Here's how the part is built. I have some questions about the finished solid (model axes, mm). A direction names the side the tool comes from. Round coordinates to 2 decimals unless told otherwise and drop trailing zeros. Write each loop counter-clockwise with the first axis right and the second up, starting at its lowest first coordinate (ties: lowest second). Pieces come first, ordered by that corner, then holes. Notation, with made-up numbers: M 31.25,28.5 L 89.25,28.5 A30 ccw 89.25,53.5 Z; hole C 3,26 d9. An arc over 180 degrees is marked long. Use a Markdown table: item, result. Add a question column.
Autodesk Inventor part; units mm, degrees
ref_plane "YZ Plane" through (0, 0, 0) normal (1, 0, 0) x (0, 1, 0)
ref_plane "XZ Plane" through (0, 0, 0) normal (0, 1, 0) x (-1, 0, 0)
ref_plane "XY Plane" through (0, 0, 0) normal (0, 0, 1) x (1, 0, 0)
sketch "main" plane through (0, 0, 0) normal (0, 0, 1) x (1, 0, 0)
  circle A0 centre (-11.2144, -104.2473) radius 2.1844
  circle A1 centre (1.4856, -104.2473) radius 2.1844
  circle A2 centre (48.9096, 6.9894) radius 2.1844
  circle A3 centre (-26.5889, 92.8058) radius 2.1844
  arc A4 (1.4856, -110.5973) -> (7.2979, -106.8047) centre (1.4856, -104.2473) ccw
  arc A5 (-17.0266, -101.6899) -> (-11.2144, -110.5973) centre (-11.2144, -104.2473) ccw
  line L0 (54.6905, 10.0319) -> (-22.1306, 97.3516)
  line L1 (55.7352, 3.2802) -> (7.2979, -106.8047)
  line L2 (-31.0925, 97.9248) -> (-34.2947, 95.1076)
  line L3 (-33.7837, 110.5973) -> (6.8178, 64.4472)
  line L4 (-17.0266, -101.6899) -> (6.006, -49.3432)
  line L5 (-34.8679, 86.1457) -> (-10.7088, 58.6849)
  arc A6 (-34.2947, 95.1076) -> (-34.8679, 86.1457) centre (-30.1004, 90.34) ccw
  arc A7 (-22.1306, 97.3516) -> (-31.0925, 97.9248) centre (-26.8981, 93.1573) ccw
  arc A8 (55.7352, 3.2802) -> (54.6905, 10.0319) centre (49.923, 5.8376) ccw
  arc A9 (6.006, -49.3432) -> (-10.7088, 58.6849) centre (-86.9901, -8.425) ccw
  line L6 (-11.2144, -110.5973) -> (1.4856, -110.5973)
  point P0 (16.4228, 13.0791)
  point P1 (-26.3249, 102.1192)
  point P2 (49.8339, -10.1318)
  dimension "d9" = 6.35
  dimension "d10" = 6.35
  dimension "d11" = 101.6
sketch "Sketch1" plane through (0, 0, 0) normal (1, 0, 0) x (0, 1, 0)
  line L0 (75.2647, -38.7566) -> (81.5639, -38.7566)
  line L1 (81.5639, -38.7566) -> (81.5639, -45.0558)
  line L2 (81.5639, -45.0558) -> (75.2647, -45.0558)
  line L3 (75.2647, -45.0558) -> (75.2647, -38.7566)
  line L4 (75.2647, -38.7566) -> (81.5639, -45.0558) construction
  line L5 (81.5639, -38.7566) -> (75.2647, -45.0558) construction
  circle A0 centre (0, 0) radius 2.1844
  circle A1 centre (0, -12.7) radius 2.1844
  circle A2 centre (111.2367, -60.124) radius 2.1844
  circle A3 centre (197.0531, 15.3746) radius 2.1844
  arc A4 (-6.35, -12.7) -> (-2.5574, -18.5123) centre (0, -12.7) ccw
  arc A5 (2.5574, 5.8123) -> (-6.35, 0) centre (0, 0) ccw
  line L6 (114.2793, -65.9049) -> (201.599, 10.9162)
  line L7 (107.5275, -66.9496) -> (-2.5574, -18.5123)
  line L8 (202.1722, 19.8781) -> (199.3549, 23.0804)
  line L9 (214.8446, 22.5693) -> (168.6945, -18.0321)
  line L10 (2.5574, 5.8123) -> (54.9042, -17.2203)
  line L11 (190.393, 23.6536) -> (162.9322, -0.5055)
  arc A6 (199.3549, 23.0804) -> (190.393, 23.6536) centre (194.5874, 18.886) ccw
  arc A7 (201.599, 10.9162) -> (202.1722, 19.8781) centre (197.4046, 15.6838) ccw
  arc A8 (107.5275, -66.9496) -> (114.2793, -65.9049) centre (110.0849, -61.1373) ccw
  arc A9 (54.9042, -17.2203) -> (162.9322, -0.5055) centre (95.8224, 75.7757) ccw
  line L12 (-6.35, 0) -> (-6.35, -12.7)
  point P0 (0, 0)
  dimension "d12" = 6.2992
  dimension "d13" = 6.2992
extrude "Extrusion1" add sketch "Sketch1" along normal blind 1.5875
properties part number "Support Gusset" material "Acetal Resin, White"
Item 1: Imagine slicing it at D-D on z = -56. List the corners of the cut face in (x, y) for me, plus the area to 3 significant figures.
Item 2: Imagine slicing it at A-A on z = -21.5. List the corners of the cut face in (x, y) for me.
Item 3: I need wall thicknesses on probe 1 along Z at (x, y) = (1.35, 0); probe 2 along Y at (x, z) = (0.25, -5); probe 3 along Y at (x, z) = (1.05, -5.5). Which ranges of each line are inside material? Lowest first, please. Write a range as from..to.
Item 4: On a 3-axis mill with a long thin cutter (end or side, diameter ignored), from which of +Z, -Z, +X, -X, +Y, -Y can I reach the whole of each face in a straight line? I mean faces 1 (the face through (0.78, 176.85, 11.74)), 2 (the face through (0.78, 199.07, 16.21)). Say none if no direction works.
Item 5: Imagine slicing it at B-B on x = 0.95. List the corners of the cut face in (y, z) for me.
Item 6: Imagine slicing it at C-C on y = 0. List the corners of the cut face in (x, z) for me, plus the area to 3 significant figures.
Item 7: For pin 1 Ø0.5 at (x, y) = (1, 79.5) entering from -Z; pin 2 Ø0.5 at (x, z) = (1, -43) entering from -Y, each with a flat end and sliding along its axis, tell me the tip position at first contact or that it passes through.
The answers:
| question | item | result |
|---|---|---|
| 1 | outline | M 0,82.64 L 1.59,82.64 L 1.59,125.54 L 0,125.54 Z |
| 1 | area | 68.1 mm² |
| 2 | outline | M 0,4.23 L 1.59,4.23 L 1.59,66.5 L 0,66.5 Z; M 0,125.15 L 1.59,125.15 L 1.59,164.75 L 0,164.75 Z |
| 3 | probe 1 | -19.64..-14.88, -10.52..-2.18, 2.18..6.35 |
| 3 | probe 2 | -6.35..27.13, 157.45..183.51 |
| 3 | probe 3 | -6.35..28.27, 156.79..182.94 |
| 4 | face 1 | +Z, +X, -X |
| 4 | face 2 | +X, -X |
| 5 | outline | M -6.35,-12.7 A6.35 ccw -2.56,-18.51 L 107.53,-66.95 A6.35 ccw 114.28,-65.9 L 201.6,10.92 A6.35 ccw 202.17,19.88 L 199.35,23.08 A6.35 ccw 190.39,23.65 L 162.93,-0.51 A101.6 cw 54.9,-17.22 L 2.56,5.81 A6.35 ccw -6.35,0 Z; hole C 0,-12.7 d4.37; hole C 0,0 d4.37; hole M 75.26,-45.06 L 81.56,-45.06 L 81.56,-38.76 L 75.26,-38.76 Z; hole C 111.24,-60.12 d4.37; hole C 197.05,15.37 d4.37 |
| 6 | outline | M 0,-19.64 L 1.59,-19.64 L 1.59,-14.88 L 0,-14.88 Z; M 0,-10.52 L 1.59,-10.52 L 1.59,-2.18 L 0,-2.18 Z; M 0,2.18 L 1.59,2.18 L 1.59,6.35 L 0,6.35 Z |
| 6 | area | 27.4 mm² |
| 7 | pin 1 | z = -54.73 |
| 7 | pin 2 | y = 52.53 |
